Could you check a few things on this drawing? It's one solid part, dimensions in mm from its lowest x, y, z. Round coordinates to 2 decimals unless told otherwise and drop trailing zeros. Loops run counter-clockwise (first coordinate to the right, second up) from the corner with the lowest first, then second, coordinate; pieces in that order, holes last. Notation, with made-up numbers: (42.5, 77) -> (54.5, 77) arc R20 ccw to (54.5, 86) -> close; hole circle Ø2 at (16, 88). An arc over 180 degrees is marked (long way). Put each result on its own line as item: value. Start each with the question number.
1. Imagine slicing it at A-A, the plane y = 83. Please give me the cut outline in (x, z).
2. I'm going to push a flat-ended pin straight in: P1, Ø8, axis at y = 52, z = 38, coming from the -X side. Where does the tip first touch, or does it pass through?
3. I need wall thicknesses on line 1 (Y direction, x = 2.25, z = 52.5); line 2 (Z direction, x = 2, y = 30); line 3 (Y direction, x = 3.25, z = 63). Which ranges of each line are inside material? Lowest first, please. Write a range as [from, to].
4. Imagine slicing it at B-B, the plane z = 17.5. Please give me the cut outline in (x, y), and give its area (3 significant figures).
5. Imagine slicing it at C-C, the plane x = 1.75. Please give me the cut outline in (y, z).
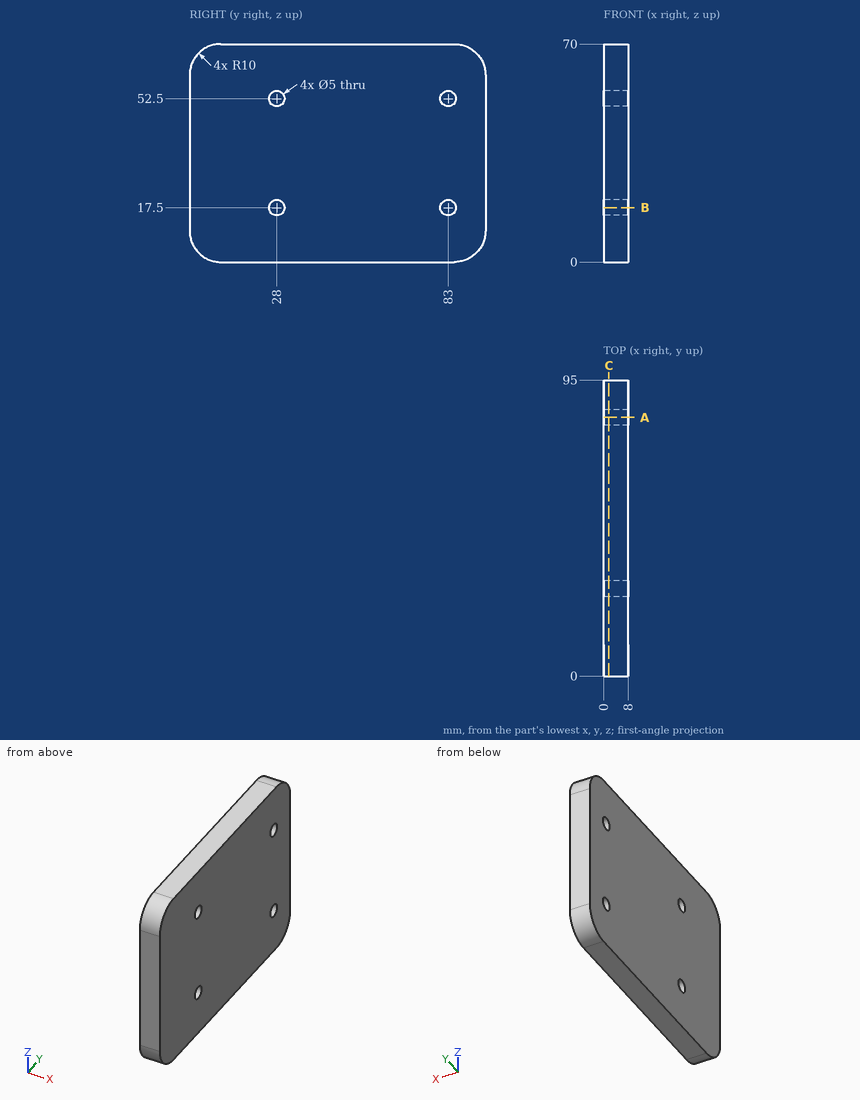
Entries:
1. outline: (0, 0) -> (8, 0) -> (8, 15) -> (0, 15) -> close; (0, 20) -> (8, 20) -> (8, 50) -> (0, 50) -> close; (0, 55) -> (8, 55) -> (8, 70) -> (0, 70) -> close
2. P1: x = 0
3. line 1: [0, 25.5], [30.5, 80.5], [85.5, 95]
3. line 2: [0, 16], [19, 51], [54, 70]
3. line 3: [0.46, 94.54]
4. outline: (0, 0) -> (8, 0) -> (8, 25.5) -> (0, 25.5) -> close; (0, 30.5) -> (8, 30.5) -> (8, 80.5) -> (0, 80.5) -> close; (0, 85.5) -> (8, 85.5) -> (8, 95) -> (0, 95) -> close
4. area: 680 mm^2
5. outline: (0, 10) arc R10 ccw to (10, 0) -> (85, 0) arc R10 ccw to (95, 10) -> (95, 60) arc R10 ccw to (85, 70) -> (10, 70) arc R10 ccw to (0, 60) -> close; hole circle Ø5 at (28, 17.5); hole circle Ø5 at (28, 52.5); hole circle Ø5 at (83, 17.5); hole circle Ø5 at (83, 52.5)
